For this review, take the finished solid that the model builds, in its own axes (mm). Face numbers are marked on the shaded views. A direction names the side the tool comes from. Give positions to 0.01 mm unless a question says otherwise; leave off trailing zeros. Write each loop counter-clockwise with the first axis right and the second up, starting at its lowest first coordinate (ties: lowest second). Pieces come first, ordered by that corner, then holes.
Q1. Insertion check: P1, Ø4, axis at x = 2.5, y = 19, coming from the +Z side; P2, Ø3.5, axis at x = 0, y = -1, coming from the +Z side; P3, Ø3.5, axis at x = 0, z = -8, coming from the -Y side. Each pin has a flat end and moves straight along its axis. Give the tip position at first contact, or say it passes through.
Q2. We need section C-C (x = -9.5). Write out the cut boundary in (y, z).
Q3. Mouldability with a two-part tool opening along Y and no side actions: class the marked faces 1, 2 and 3 as released by +Y, released by -Y, zero draft, split by the parting line, or undercut.
Q4. We need section D-D (z = -8). Write out the cut boundary in (x, y).
Q5. Machinability: for the marked faces 4, 5, 6, 7 and 8, which of the approach directions +Z, -Z, +X, -X, +Y, -Y give a long, thin tool a straight path to every point of the face, cutting with its end or side? Answer none if there is none.
Q6. We need section B-B (y = 3). Write out the cut boundary in (x, z), then the cut area to 3 significant figures.
Q7. For line 1 (X direction, y = 27.2, z = 0); line 2 (X direction, y = -1, z = 6.5); line 3 (X direction, y = 6, z = 0), list the stretches that pass through material, from the lowest coordinate up.
Q8. We need section A-A (z = 8). Write out the cut boundary in (x, y).
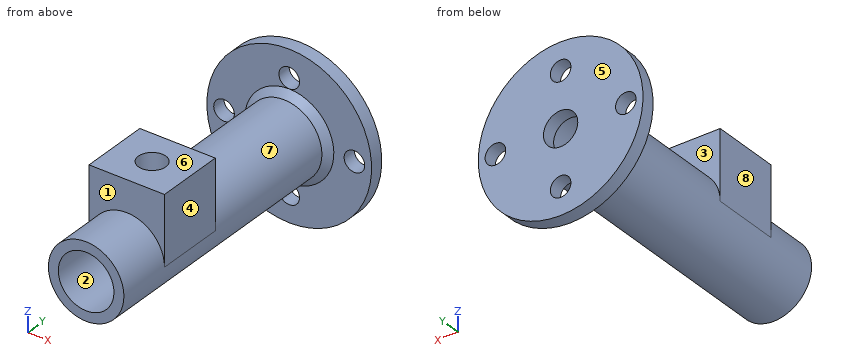
```python
from build123d import *

# Parameters (mm, degrees)
SKETCH1_R                = 16
SKETCH1_R_2              = 14
BOSS_EXTRUDE1_DEPTH      = 26
SKETCH2_R                = 16
BOSS_EXTRUDE2_DEPTH      = 2
SKETCH3_R                = 1.5
CUT_EXTRUDE1_DEPTH       = 2
CUT_EXTRUDE2_DEPTH       = 26
SKETCH5_R                = 2.5
CUT_EXTRUDE3_DEPTH       = 10
SKETCH9_R                = 22.610796359
SKETCH9_R_2              = 12
CUT_EXTRUDE4_DEPTH       = 44
SKETCH10_R               = 5.5
SKETCH10_R_2             = 4.05
BOSS_EXTRUDE3_DEPTH      = 40
BOSS_EXTRUDE4_DEPTH      = 6
BOSS_EXTRUDE4_DEPTH_BACK = 4.05
SKETCH13_W               = 11
SKETCH13_H               = 10
SKETCH13_R               = 2
CUT_EXTRUDE5_START       = -33
SKETCH14_R               = 4.05
CUT_EXTRUDE5_DEPTH       = 33
CUT_EXTRUDE6_START       = -10
SKETCH15_R               = 2
CUT_EXTRUDE6_DEPTH       = 10
CHAMFER3_SIZE            = 1


with BuildPart() as part:
    # Sketch1 → Boss-Extrude1 (new body)
    with BuildSketch(Plane(origin=(0, 0, 0), x_dir=(1, 0, 0), z_dir=(0, 1, 0))):
        with Locations(Location((0, 0, 0), (0, 0, 90))):
            Circle(SKETCH1_R)
        with Locations(Location((0, 0, 0), (0, 0, 90))):
            Circle(SKETCH1_R_2, mode=Mode.SUBTRACT)
    extrude(amount=BOSS_EXTRUDE1_DEPTH)

    # Sketch2 → Boss-Extrude2 (add)
    with BuildSketch(Plane(origin=(0, 26, 0), x_dir=(1, 0, 0), z_dir=(0, 1, 0))):
        with Locations(Location((0, 0, 0), (0, 0, 90))):
            Circle(SKETCH2_R)
    extrude(amount=BOSS_EXTRUDE2_DEPTH)

    # Sketch3 → Cut-Extrude1 (cut)
    with BuildSketch(Plane.XZ.offset(-26)):
        with Locations(Location((0, 8, 0), (0, 0, 270))):
            Circle(SKETCH3_R)
        with Locations(Location((9.5, 0, 0), (0, 0, 270))):
            Circle(SKETCH3_R)
        with Locations(Location((-9.5, 0, 0), (0, 0, 270))):
            Circle(SKETCH3_R)
        with Locations(Location((0, -8, 0), (0, 0, 270))):
            Circle(SKETCH3_R)
    extrude(amount=-CUT_EXTRUDE1_DEPTH, mode=Mode.SUBTRACT)

    # Sketch4 → Cut-Extrude2 (cut)
    with BuildSketch(Plane.XZ):
        Polygon((-0.813172798, -5.550788232), (5.550788232, 0.813172798), (16.15738995, -9.793428919), (9.793428919, -16.15738995), align=None)
    extrude(amount=-CUT_EXTRUDE2_DEPTH, mode=Mode.SUBTRACT)

    # Sketch5 → Cut-Extrude3 (cut)
    with BuildSketch(Plane.XZ.offset(-26)):
        with Locations(Location((0, 0, 0), (0, 0, 270))):
            Circle(SKETCH5_R)
    extrude(amount=-CUT_EXTRUDE3_DEPTH, mode=Mode.SUBTRACT)

    # Sketch9 → Cut-Extrude4 (cut)
    with BuildSketch(Plane.XZ):
        Circle(SKETCH9_R)
        with Locations(Location((0, 0, 0), (0, 0, 90))):
            Circle(SKETCH9_R_2, mode=Mode.SUBTRACT)
    extrude(amount=-CUT_EXTRUDE4_DEPTH, mode=Mode.SUBTRACT)

    # Sketch10 → Boss-Extrude3 (add)
    with BuildSketch(Plane.XZ.offset(-26)):
        with Locations(Location((0, 0, 0), (0, 0, 90))):
            Circle(SKETCH10_R)
        with Locations(Location((0, 0, 0), (0, 0, 270))):
            Circle(SKETCH10_R_2, mode=Mode.SUBTRACT)
    extrude(amount=BOSS_EXTRUDE3_DEPTH)

    # Sketch13 → Boss-Extrude4 (add, two sides: drawn at the far end of the back side and taken through both)
    with BuildSketch(Plane.XY.offset(4.05).offset(-BOSS_EXTRUDE4_DEPTH_BACK)):
        with Locations((0, -1)):
            Rectangle(SKETCH13_W, SKETCH13_H)
        with Locations((0, -1)):
            Circle(SKETCH13_R, mode=Mode.SUBTRACT)
    extrude(amount=BOSS_EXTRUDE4_DEPTH + BOSS_EXTRUDE4_DEPTH_BACK)

    # Sketch14 → Cut-Extrude5 (cut)
    with BuildSketch(Plane.XZ.offset(14).offset(CUT_EXTRUDE5_START)):
        with Locations(Location((0, 0, 0), (0, 0, 270))):
            Circle(SKETCH14_R)
    extrude(amount=CUT_EXTRUDE5_DEPTH, mode=Mode.SUBTRACT)

    # Sketch15 → Cut-Extrude6 (cut)
    with BuildSketch(Plane.XY.offset(10.05).offset(CUT_EXTRUDE6_START)):
        with Locations((0, -1)):
            Circle(SKETCH15_R)
    extrude(amount=CUT_EXTRUDE6_DEPTH, mode=Mode.SUBTRACT)

    # Chamfer3
    chamfer3_edges = [part.edges().sort_by_distance(p)[0] for p in [
        (0, 26, -5.5),
    ]]
    chamfer(chamfer3_edges, length=CHAMFER3_SIZE - 0.0001)  # a hair under: the kernel refuses the full size


solid = part.part
```
Computed:
1. P1: stops at z = 5.48
1. P2: stops at z = -3.65
1. P3: stops at y = 25.75
2. outline: (26, -7.33) - (28, -7.33) - (28, -1.5) - (26, -1.5) - close; (26, 1.5) - (28, 1.5) - (28, 7.33) - (26, 7.33) - close
3. face 1: released by -Y
3. face 2: zero draft
3. face 3: undercut
4. outline: (-8.94, 26) - (-1.5, 26) - (-1.5, 28) - (-8.94, 28) - close; (1.5, 26) - (8.94, 26) - (8.94, 28) - (1.5, 28) - close
5. face 4: +Z, -Z, +X, -Y
5. face 5: +Z, -Z, +X, -X, +Y
5. face 6: +Z, +X, -X, -Y
5. face 7: none
5. face 8: +Z, -Z, -X, -Y
6. outline: (-5.5, 0) arc R5.5 ccw to (5.5, 0) - (5.5, 10.05) - (-5.5, 10.05) - close; hole circle Ø8.1 at (0, 0)
6. area: 107 mm2
7. line 1: x = -12 to -11, -8 to -2.5, 2.5 to 8, 11 to 12
7. line 2: x = -5.5 to -2, 2 to 5.5
7. line 3: x = -5.5 to -4.05, 4.05 to 5.5
8. outline: (-8.94, 26) - (-1.5, 26) - (-1.5, 28) - (-8.94, 28) - close; (-5.5, -6) - (5.5, -6) - (5.5, 4) - (-5.5, 4) - close; (1.5, 26) - (8.94, 26) - (8.94, 28) - (1.5, 28) - close; hole circle Ø4 at (0, -1)
